Can you work these out from the model? Positions are in its coordinate system, mm. Coordinates: 2 decimals unless noted, no trailing zeros. Order: outer loops, then holes, each group sorted by start corner. A loop starts at its lowest first (then second) coordinate and runs counter-clockwise, first axis right, second up. Notation, with made-up numbers: (35.25, 81.5) -> (59.25, 81.5) arc R23 cw to (59.25, 106.5) -> close; hole circle Ø1 at (86.5, 87). An arc over 180 degrees is marked (long way). Answer as a JSON object with one key per item and string values. Group by question number.
(1) I want a section at A-A, the plane x = 22.5. List the corners of the cut face in (y, z) for me.
(2) For pin 1 (4.5 mm diameter, centred on x = 29.46, y = -20.15, fed in from +Z); pin 2 (1 mm diameter, centred on x = 24.5, z = 2, fed in from +Y); pin 3 (1.5 mm diameter, centred on x = 20, z = 1.5, fed in from +Y); pin 4 (1 mm diameter, centred on y = -35.5, z = 2.5, fed in from -X), each with a flat end and sliding along its axis, tell me the tip position at first contact or that it passes through.
(3) I need wall thicknesses on line 1 (X direction, y = -24, z = 4.05); line 2 (Y direction, x = 30, z = 3); line 3 (Y direction, x = 24.5, z = 3.05). Which ranges of each line are inside material? Lowest first, please.
(4) I want a section at B-B, the plane y = -25. List the corners of the cut face in (x, z) for me.
(5) I want a section at C-C, the plane z = 3.9. List the corners of the cut face in (x, y) for me, plus the area to 3 significant figures.
(6) If we mould it in two halves opening along X, with no side actions, what happens to faces 1 (the cylindrical face through (24.38, -20.57, 2.25)), 2 (the flat face through (14, -22, 0)), 3 (the cylindrical face through (20.05, -43.836, 2.254))? For each: pulls with the +X half, pulls with the -X half, needs draft (parallel to the pull), parting line crosses it, or undercut.
(7) I want a section at D-D, the plane x = 17.5. List the corners of the cut face in (y, z) for me.
from build123d import *

# Parameters (mm, degrees)
F0_R     = 3.251044
F0_R_2   = 2.532183
F1_DEPTH = 4.572


with BuildPart() as f1:
    # F0 (on Top) → F1 (new body)
    with BuildSketch(Plane.XY):
        with BuildLine():
            ThreePointArc((26.297173, -6.489626), (20.14867, -1.814141), (12.640465, 0))
            ThreePointArc((12.640465, 0), (0.511468, -8.706083), (5.432757, -22.801805))
            ThreePointArc((5.432757, -22.801805), (0.511468, -36.897527), (12.640465, -45.603611))
            ThreePointArc((12.640465, -45.603611), (20.14867, -43.78947), (26.297173, -39.113984))
            ThreePointArc((26.297173, -39.113984), (31.520039, -33.141343), (37.551314, -27.986296))
            ThreePointArc((37.551314, -27.986296), (34.86808, -22.801805), (37.551314, -17.617315))
            ThreePointArc((37.551314, -17.617315), (31.520039, -12.462268), (26.297173, -6.489626))
        make_face()
        with Locations((22.630094, -23.30761)):
            Circle(F0_R, mode=Mode.SUBTRACT)
        with Locations((29.45845, -20.146335)):
            Circle(F0_R_2, mode=Mode.SUBTRACT)
    extrude(amount=F1_DEPTH)


solid = f1.part
Computed values:
{
 "1": {"outline": "(-42.46, 0) -> (-26.56, 0) -> (-26.56, 4.57) -> (-42.46, 4.57) -> close; (-20.06, 0) -> (-3.15, 0) -> (-3.15, 4.57) -> (-20.06, 4.57) -> close"},
 "2": {"pin 1": "passes through", "pin 2": "stops at y = -4.26", "pin 3": "stops at y = -1.42", "pin 4": "stops at x = 0.07"},
 "3": {"line 1": "x = 3.92 to 19.45, 25.81 to 34.98", "line 2": "y = -34.71 to -22.62, -17.67 to -10.9", "line 3": "y = -40.92 to -25.97, -20.65 to -4.68"},
 "4": {"outline": "(2.96, 0) -> (19.85, 0) -> (19.85, 4.57) -> (2.96, 4.57) -> close; (25.41, 0) -> (35.26, 0) -> (35.26, 4.57) -> (25.41, 4.57) -> close"},
 "5": {"outline": "(5.43, -22.8) arc R12.47 ccw to (12.64, -45.6) arc R18.83 ccw to (26.3, -39.11) arc R54.75 cw to (37.55, -27.99) arc R6.35 cw to (37.55, -17.62) arc R54.75 cw to (26.3, -6.49) arc R18.83 ccw to (12.64, 0) arc R12.47 ccw to start; hole circle Ø6.5 at (22.63, -23.31); hole circle Ø5.06 at (29.46, -20.15)", "area": "1,200 mm2"},
 "6": {"face 1": "undercut", "face 2": "needs draft", "face 3": "pulls with the +X half"},
 "7": {"outline": "(-44.81, 0) -> (-0.79, 0) -> (-0.79, 4.57) -> (-44.81, 4.57) -> close"}
}
